Input: dimensioned drawing with shaded views. Units: mm. Origin: part minimum x, y, z. A direction names the side the tool comes from. Give positions to 0.01 mm unless a question says otherwise; leave off trailing zeros. Write each loop counter-clockwise with the first axis right and the second up, starting at its lowest first coordinate (ties: lowest second). Pieces come first, ordered by that corner, then holes.
Q1. Mould query, pull axis X, two halves, no side actions, for the marked faces 3, 4 and 5. Classes: +X half, -X half, draft (parallel to the pull), parting line (faces both ways), or undercut.
Q2. Line query: line 1 (X direction, y = 15.5, z = 4); line 2 (X direction, y = 14, z = 5); line 3 (Z direction, x = 23, y = 24). Output: solid intervals per line, ascending.
Q3. Section A-A (z = 5). Return the cut outline in (x, y).
Q4. Pin query (flat end, axial travel): pin 1 Ø1.9 at (y, z) = (16, 3) entering from +X; pin 2 Ø4 at (x, y) = (17.5, 12.5) entering from -Z; pin 3 Ø1 at (y, z) = (15, 17.5) entering from -X (1 decimal); pin 4 Ø1 at (x, z) = (7, 21.5) entering from +Y. Return the tip coordinate at first contact, or that it passes through.
Q5. Reachability of the marked faces 1 and 2 from +Z, -Z, +X, -X, +Y, -Y: full face, straight path, thin tool, end or side. Return the list, or none.
Q6. Section D-D (z = 29.5). Return the cut outline in (x, y) (1 decimal), plus the area to 3 significant figures.
Q7. Section C-C (x = 6.5). Return the cut outline in (y, z) (1 decimal).
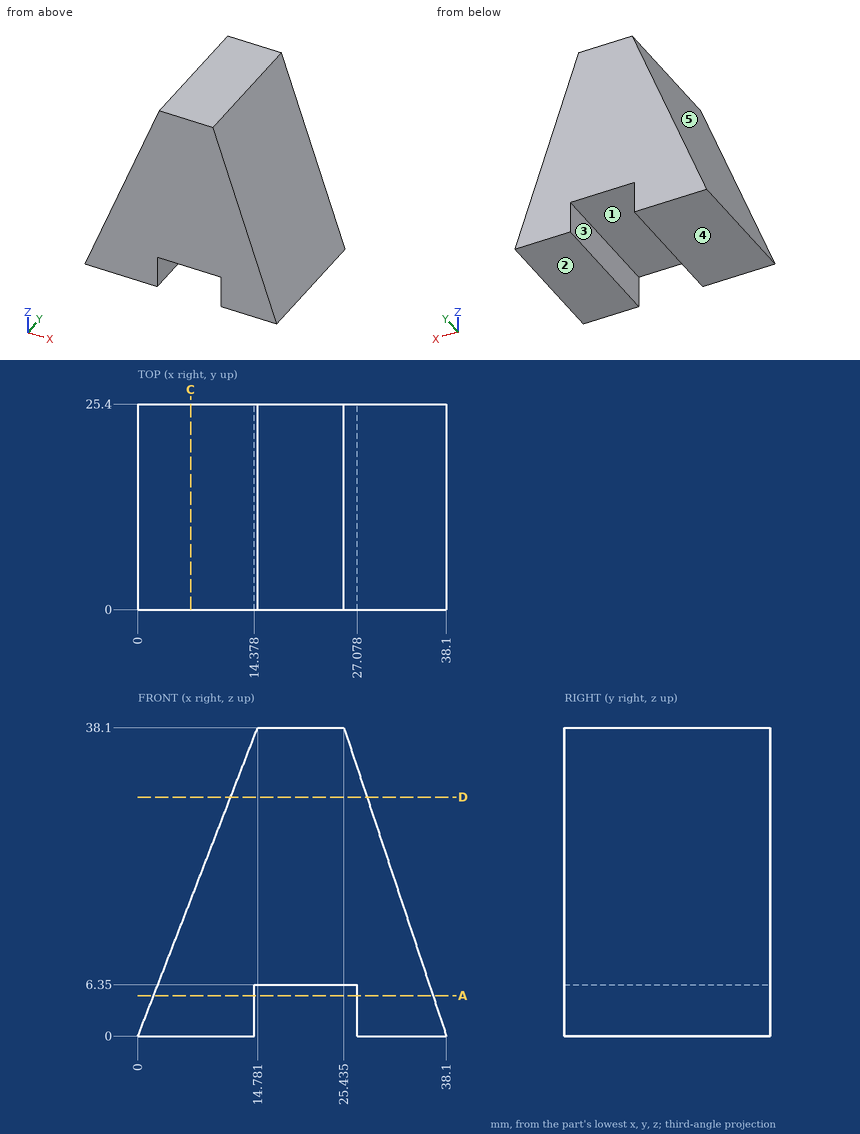
Computed:
1. face 3: undercut
1. face 4: draft
1. face 5: -X half
2. line 1: x = 1.55 to 14.38, 27.08 to 36.77
2. line 2: x = 1.94 to 14.38, 27.08 to 36.44
2. line 3: z = 6.35 to 38.1
3. outline: (1.94, 0) - (14.38, 0) - (14.38, 25.4) - (1.94, 25.4) - close; (27.08, 0) - (36.44, 0) - (36.44, 25.4) - (27.08, 25.4) - close
4. pin 1: stops at x = 37.42
4. pin 2: stops at z = 6.35
4. pin 3: stops at x = 6.6
4. pin 4: passes through
5. face 1: -Z, +Y, -Y
5. face 2: -Z, +X, -X, +Y, -Y
6. outline: (11.4, 0) - (28.3, 0) - (28.3, 25.4) - (11.4, 25.4) - close
6. area: 428 mm2
7. outline: (0, 0) - (25.4, 0) - (25.4, 16.8) - (0, 16.8) - close
